Geometry: final body of the model. Coordinates: model frame, mm. A direction names the side the tool comes from. Give positions to 0.01 mm unless a question says otherwise; leave off trailing zeros. Loops run counter-clockwise (first coordinate to the right, second up) from the corner with the lowest first, then second, coordinate; pieces in that order, holes last.
1. Material intervals for line 1 along Y through (x, z) = (687, 11); line 2 along Y through (x, z) = (193.5, 14); line 3 along X through (y, z) = (40, 17.75), sorted ascending.
2. Section A-A, the plane x = 799. Output: boundary loops of the cut face in (y, z).
3. Access query for faces 5 (the face through (228.6, 113, 10)), 6 (the face through (571, 96, 0)). Directions: +Z, -Z, +X, -X, +Y, -Y. A direction counts if a zero-diameter tool reaches every point of the face in a straight line with its end or side. Return the directions, or none.
4. Draft query along Y for faces 1 (the face through (635, 75, 10)), 2 (the face through (549.792, 277.996, 9.392)), 3 (the face through (0, 58, 9)), 4 (the face through (660.4, 77, 10)). Return one class per face: +Y half, -Y half, draft (parallel to the pull), parting line (faces both ways), or undercut.
5. First-contact query: P1, Ø1.5, axis at y = 82, z = 3.5, coming from the -X side; P2, Ø5, axis at y = 152.5, z = 9.5, coming from the -X side; P3, Ø14.5, axis at x = 963.57, y = 244.87, coming from the -Z side; P4, Ø5, axis at x = 316.5, z = 3, coming from the +Y side. Flat tips, straight axial feed; report the tip coordinate or a pass-through.
6. Section B-B, the plane z = 9. State how many separate pieces and enclosed holes the cut face has, then the cut area to 3 significant figures.
7. Section C-C, the plane y = 297.5. Output: boundary loops of the cut face in (x, z), then the cut area to 3 significant figures.
from build123d import *

# Parameters (mm, degrees)
BOSS_EXTRUDE1_DEPTH = 19.05
SKETCH8_R           = 6.35
CUT_EXTRUDE3_DEPTH  = 1187.240784438
SKETCH10_R          = 7.9375
CUT_EXTRUDE5_DEPTH  = 1187.240784438
CUT_EXTRUDE6_DEPTH  = 1187.240784438
SKETCH13_R          = 7.9375
CUT_EXTRUDE7_DEPTH  = 1187.240784438


with BuildPart() as part:
    # Sketch1 → Boss-Extrude1 (new body)
    with BuildSketch(Plane.XY):
        Polygon((-10.620091868, 219.094223225), (1126.118434538, 338.57025674), (1136.738526406, 237.526832171), (1136.738526406, 0), (0, 0), (0, 118.050798656), align=None)
    extrude(amount=BOSS_EXTRUDE1_DEPTH)

    # Sketch8 → Cut-Extrude3 (cut, through all)
    with BuildSketch(Plane.XY.offset(19.05)):
        with Locations((104.703615638, 154.595502408)):
            Circle(SKETCH8_R)
    extrude(amount=-CUT_EXTRUDE3_DEPTH, mode=Mode.SUBTRACT)

    # Sketch10 → Cut-Extrude5 (cut, through all)
    with BuildSketch(Plane.XY.offset(19.05)):
        with Locations((963.572724478, 244.866283286)):
            Circle(SKETCH10_R)
        with Locations((966.199929442, 214.837193133)):
            Circle(SKETCH10_R)
        with Locations((967.777533852, 184.73470776)):
            Circle(SKETCH10_R)
        with Locations((968.303615638, 154.595502408)):
            Circle(SKETCH10_R)
        with Locations((959.899119803, 274.785392397)):
            Circle(SKETCH10_R)
    extrude(amount=-CUT_EXTRUDE5_DEPTH, mode=Mode.SUBTRACT)

    # Sketch12 → Cut-Extrude6 (cut, through all)
    with BuildSketch(Plane.XY.offset(19.05)):
        with BuildLine():
            Line((844.55, 50.8), (666.75, 50.8))
            ThreePointArc((666.75, 50.8), (662.259871939, 52.659871939), (660.4, 57.15))
            Line((660.4, 57.15), (660.4, 96.816443106))
            ThreePointArc((660.4, 96.816443106), (662.031030358, 101.065422457), (666.086244258, 103.131657142))
            Line((666.086244258, 103.131657142), (843.886244258, 121.819190172))
            ThreePointArc((843.886244258, 121.819190172), (848.79897935, 120.222945778), (850.9, 115.503976137))
            Line((850.9, 115.503976137), (850.9, 57.15))
            ThreePointArc((850.9, 57.15), (849.040128061, 52.659871939), (844.55, 50.8))
        make_face()
        with BuildLine():
            Line((444.5, 57.15), (444.5, 74.124438713))
            ThreePointArc((444.5, 74.124438713), (446.131030358, 78.373418063), (450.186244258, 80.439652748))
            Line((450.186244258, 80.439652748), (627.986244258, 99.127185778))
            ThreePointArc((627.986244258, 99.127185778), (632.89897935, 97.530941385), (635, 92.811971743))
            Line((635, 92.811971743), (635, 57.15))
            ThreePointArc((635, 57.15), (633.140128061, 52.659871939), (628.65, 50.8))
            Line((628.65, 50.8), (450.85, 50.8))
            ThreePointArc((450.85, 50.8), (446.359871939, 52.659871939), (444.5, 57.15))
        make_face()
        with BuildLine():
            Line((843.886244258, 206.74681701), (666.086244258, 188.05928398))
            ThreePointArc((666.086244258, 188.05928398), (662.031030358, 185.993049294), (660.4, 181.744069944))
            Line((660.4, 181.744069944), (660.4, 135.126308558))
            ThreePointArc((660.4, 135.126308558), (662.50102065, 130.407338916), (667.413755742, 128.811094522))
            Line((667.413755742, 128.811094522), (845.213755742, 147.498627552))
            ThreePointArc((845.213755742, 147.498627552), (849.268969642, 149.564862238), (850.9, 153.813841588))
            Line((850.9, 153.813841588), (850.9, 200.431602974))
            ThreePointArc((850.9, 200.431602974), (848.79897935, 205.150572616), (843.886244258, 206.74681701))
        make_face()
        with BuildLine():
            Line((627.986244258, 184.054812616), (450.186244258, 165.367279586))
            ThreePointArc((450.186244258, 165.367279586), (446.131030358, 163.301044901), (444.5, 159.05206555))
            Line((444.5, 159.05206555), (444.5, 112.434304164))
            ThreePointArc((444.5, 112.434304164), (446.60102065, 107.715334522), (451.513755742, 106.119090128))
            Line((451.513755742, 106.119090128), (629.313755742, 124.806623159))
            ThreePointArc((629.313755742, 124.806623159), (633.368969642, 126.872857844), (635, 131.121837194))
            Line((635, 131.121837194), (635, 177.73959858))
            ThreePointArc((635, 177.73959858), (632.89897935, 182.458568222), (627.986244258, 184.054812616))
        make_face()
        with BuildLine():
            Line((412.75, 50.8), (234.95, 50.8))
            ThreePointArc((234.95, 50.8), (231.455726331, 54.115941899), (234.584247692, 57.778969777))
            Line((234.584247692, 57.778969777), (412.086244258, 76.435181385))
            ThreePointArc((412.086244258, 76.435181385), (416.99897935, 74.838936991), (419.1, 70.119967349))
            Line((419.1, 70.119967349), (419.1, 57.15))
            ThreePointArc((419.1, 57.15), (417.240128061, 52.659871939), (412.75, 50.8))
        make_face()
        with BuildLine():
            Line((234.286244258, 142.675275192), (412.086244258, 161.362808222))
            ThreePointArc((412.086244258, 161.362808222), (416.99897935, 159.766563828), (419.1, 155.047594187))
            Line((419.1, 155.047594187), (419.1, 108.4298328))
            ThreePointArc((419.1, 108.4298328), (417.468969642, 104.18085345), (413.413755742, 102.114618765))
            Line((413.413755742, 102.114618765), (235.613755742, 83.427085734))
            ThreePointArc((235.613755742, 83.427085734), (230.70102065, 85.023330128), (228.6, 89.74229977))
            Line((228.6, 89.74229977), (228.6, 136.360061156))
            ThreePointArc((228.6, 136.360061156), (230.231030358, 140.609040507), (234.286244258, 142.675275192))
        make_face()
    extrude(amount=-CUT_EXTRUDE6_DEPTH, mode=Mode.SUBTRACT)

    # Sketch13 → Cut-Extrude7 (cut, through all)
    with BuildSketch(Plane.XY.offset(19.05)):
        with Locations((76.2, 76.2)):
            Circle(SKETCH13_R)
    extrude(amount=-CUT_EXTRUDE7_DEPTH, mode=Mode.SUBTRACT)


solid = part.part
Answers below:
1. line 1: y = 0 to 50.8, 105.33 to 130.87, 190.26 to 292.42
1. line 2: y = 0 to 240.55
1. line 3: x = 0 to 1136.74
2. outline: (0, 0) - (50.8, 0) - (50.8, 19.05) - (0, 19.05) - close; (117.1, 0) - (142.64, 0) - (142.64, 19.05) - (117.1, 19.05) - close; (202.03, 0) - (304.19, 0) - (304.19, 19.05) - (202.03, 19.05) - close
3. face 5: +Z, -Z
3. face 6: -Z, +X, -X, +Y, -Y
4. face 1: undercut
4. face 2: +Y half
4. face 3: draft
4. face 4: undercut
5. P1: stops at x = 0
5. P2: stops at x = -3.88
5. P3: passes through
5. P4: stops at y = 253.74
6. separate pieces: 1
6. enclosed holes: 13
6. area: 261,000 mm2
7. outline: (735.36, 0) - (1130.44, 0) - (1130.44, 19.05) - (735.36, 19.05) - close
7. area: 7,530 mm2
